Here's how the part is built. I have some questions about the finished solid (model axes, mm). A direction names the side the tool comes from. Round coordinates to 2 decimals unless told otherwise and drop trailing zeros. Write each loop counter-clockwise with the first axis right and the second up, starting at its lowest first coordinate (ties: lowest second). Pieces come first, ordered by that corner, then holes. Notation, with made-up numbers: (44.5, 85.25) - (79.5, 85.25) arc R21 cw to (79.5, 105.25) - close; hole circle Ø11 at (43.5, 1). An arc over 180 degrees is marked (long way). Return JSON: item names as keys, results as strings. Group by question number.
```python
from build123d import *

# Parameters (mm, degrees)
SM_BASE_FLANGE_1_DEPTH = 148.5
CUT_EXTRUDE_1_DEPTH    = 151.802022533


# Sheet-metal steps are written as plain solids
with BuildPart() as part:
    # Sketch 2 → Базовая кромка1 (new body)
    with BuildSketch(Plane.XY):
        with BuildLine():
            Line((0, -20), (0, -4.5))
            ThreePointArc((0, -4.5), (1.318019485, -1.318019485), (4.5, 0))
            Line((4.5, 0), (20, 0))
            Line((20, 0), (20, -3))
            Line((20, -3), (4.5, -3))
            ThreePointArc((4.5, -3), (3.439339828, -3.439339828), (3, -4.5))
            Line((3, -4.5), (3, -20))
            Line((3, -20), (0, -20))
        make_face()
    extrude(amount=SM_BASE_FLANGE_1_DEPTH)

    # Эскиз10 → Вырез-Вытянуть1 (cut, through all)
    with BuildSketch(Plane(origin=(3, 0, 0), x_dir=(0, 0, -1), z_dir=(1, 0, 0))):
        with BuildLine():
            Line((-140, -25.5), (-140, -14.5))
            ThreePointArc((-140, -14.5), (-135, -9.5), (-130, -14.5))
            Line((-130, -14.5), (-130, -25.5))
            ThreePointArc((-130, -25.5), (-135, -30.5), (-140, -25.5))
        make_face()
    extrude(amount=-CUT_EXTRUDE_1_DEPTH, mode=Mode.SUBTRACT)

    # Зеркальное отражение1: part across plane


with BuildPart() as part_1:
    add(part.part)
    add(part.part.mirror(Plane(origin=(4.5, -4.5, 0), x_dir=(1, 0, 0), z_dir=(0, 0, 1))))


solid = part_1.part
```
1) Imagine slicing it at C-C (y = -7). Please give me the cut outline in (x, z).
2) Imagine slicing it at A-A (z = 135). Please give me the cut outline in (x, y), plus the area to 3 significant figures.
3) Imagine slicing it at D-D (z = 74). Please give me the cut outline in (x, y), plus the area to 3 significant figures.
4) Imagine slicing it at B-B (x = 17). Please give me the cut outline in (y, z), plus the area to 3 significant figures.
5) I need wall thicknesses on line 1 along Z through (x, y) = (2.75, -16.5); line 2 along X through (y, z) = (-19, 102); line 3 along Y through (x, z) = (9.5, -102). Which ranges of each line are inside material? Lowest first, please.
6) For faces 1 (the flat face through (3, -12, 2)), 2 (the cylindrical face through (1.283, -1.353, 2.079)), which set-ups out of +Z, -Z, +X, -X, +Y, -Y let a thin tool reach every point of the face, with its end or its side?
7) If we mould it in two halves opening along Z, with no side actions, what happens to faces 3 (the flat face through (12, -3, 2)), 4 (the flat face through (2.6, -5.5, 148.5)), 5 (the cylindrical face through (1.5, -9.5, 135.1))? For each: released by +Z, released by -Z, zero draft, split by the parting line, or undercut.
8) Will these pins go through, and if not, where does the flat tip stop? pin 1 Ø1 at (y, z) = (-3, -72) entering from -X; pin 2 Ø1 at (x, z) = (15.5, 29) entering from -Y.
Results found:
{
 "1": {"outline": "(0, -148.5) - (3, -148.5) - (3, 148.5) - (0, 148.5) - close"},
 "2": {"outline": "(0, -9.5) - (3, -9.5) - (3, -4.5) arc R1.5 cw to (4.5, -3) - (20, -3) - (20, 0) - (4.5, 0) arc R4.5 ccw to (0, -4.5) - close", "area": "75.6 mm²"},
 "3": {"outline": "(0, -20) - (3, -20) - (3, -4.5) arc R1.5 cw to (4.5, -3) - (20, -3) - (20, 0) - (4.5, 0) arc R4.5 ccw to (0, -4.5) - close", "area": "107 mm²"},
 "4": {"outline": "(-3, -148.5) - (0, -148.5) - (0, 148.5) - (-3, 148.5) - close", "area": "891 mm²"},
 "5": {"line 1": "z = -148.5 to -140, -130 to 130, 140 to 148.5", "line 2": "x = 0 to 3", "line 3": "y = -3 to 0"},
 "6": {"face 1": "+Z, -Z, +X, -Y", "face 2": "+Z, -Z, -X, +Y"},
 "7": {"face 3": "zero draft", "face 4": "released by +Z", "face 5": "undercut"},
 "8": {"pin 1": "stops at x = 0.11", "pin 2": "stops at y = -3"}
}
